Verification items for the finished model (mm, model axes). Face numbers are marked on the shaded views. A direction names the side the tool comes from. Coordinates: 2 decimals unless noted, no trailing zeros. Loops run counter-clockwise (first coordinate to the right, second up) from the corner with the lowest first, then second, coordinate; pieces in that order, holes last. Notation, with made-up numbers: (-4, 86.25) -> (23, 86.25) arc R22 ccw to (23, 92.25) -> close; hole circle Ø1 at (-23.5, -7.75). An arc over 180 degrees is marked (long way). Use CSV: the item, a comma, the result in double quotes. Start each with the question number.
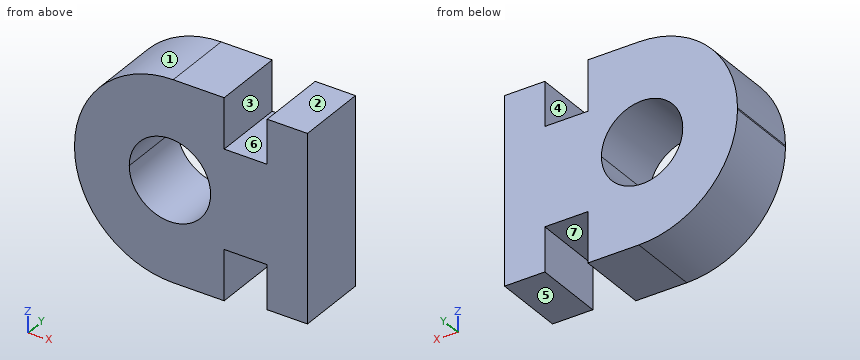
```python
from build123d import *

# Parameters (mm, degrees)
F1_DEPTH = 28.956
F2_R     = 39.858666


with BuildPart() as f1:
    # F0 (on Front) → F1 (new body)
    with BuildSketch(Plane.XZ):
        with BuildLine():
            Line((0, -37.671965), (0, 0))
            Line((0, 0), (-39.146767, 0))
            ThreePointArc((-39.146767, 0), (-55.584025, -16.437258), (-72.021282, 0))
            Line((-72.021282, 0), (-94.127469, 0))
            Line((-94.127469, 0), (-94.127469, -40.149245))
            Line((-94.127469, -40.149245), (-65.204445, -40.149245))
            Line((-65.204445, -40.149245), (-55.504855, -40.149245))
            Line((-55.504855, -40.149245), (-33.65957, -40.149245))
            Line((-33.65957, -40.149245), (-33.65957, -19.839078))
            Line((-33.65957, -19.839078), (-16.272509, -19.839078))
            Line((-16.272509, -19.839078), (-16.272509, -36.780316))
            Line((-16.272509, -36.780316), (-16.272509, -37.671965))
            Line((-16.272509, -37.671965), (0, -37.671965))
        make_face()
        with BuildLine():
            Line((0, 0), (0, 37.671965))
            Line((0, 37.671965), (-16.272509, 37.671965))
            Line((-16.272509, 37.671965), (-16.272509, 36.780316))
            Line((-16.272509, 36.780316), (-16.272509, 19.839078))
            Line((-16.272509, 19.839078), (-33.65957, 19.839078))
            Line((-33.65957, 19.839078), (-33.65957, 40.149245))
            Line((-33.65957, 40.149245), (-55.504855, 40.149245))
            Line((-55.504855, 40.149245), (-65.204445, 40.149245))
            Line((-65.204445, 40.149245), (-94.127469, 40.149245))
            Line((-94.127469, 40.149245), (-94.127469, 0))
            Line((-94.127469, 0), (-72.021282, 0))
            ThreePointArc((-72.021282, 0), (-55.584025, 16.437258), (-39.146767, 0))
            Line((-39.146767, 0), (0, 0))
        make_face()
    extrude(amount=F1_DEPTH)

    # F2
    f2_edges = [f1.edges().sort_by_distance(p)[0] for p in [
        (-94.127469, -14.478, 40.149245),
        (-94.127469, -14.478, -40.149245),
    ]]
    fillet(f2_edges, radius=F2_R)


solid = f1.part
```
1. Cross-section at A-A, the plane z = -28.5. Record the boundary of the cut face in (x, y), plus the area to 3 significant figures.
2. Cross-section at B-B, the plane y = -3.5. Record the boundary of the cut face in (x, z).
3. Release check for a two-part mould opening along X. For the marked faces 1, 2, 3 and 4 record: released by +X, released by -X, zero draft, split by the parting line, or undercut.
4. Scan lines: line 1 (X direction, y = -16.5, z = -25); line 2 (X direction, y = -6.75, z = 15); line 3 (Z direction, x = -45.5, y = -23.5). Record each from-to range of solid material in increasing order.
5. Cross-section at D-D, the plane x = -28.5. Record the boundary of the cut face in (y, z).
6. Depth check by flat-ended pin: pin 1 (3 mm diameter, centred on y = -20.5, z = -28.5, fed in from -X); pin 2 (8 mm diameter, centred on y = -17.5, z = -16, fed in from -X); pin 3 (1.5 mm diameter, centred on x = -76.5, y = -8.5, fed in from +Z). Enter the tip coordinate at first touch or a pass-through.
7. Set-up check for the marked faces 5, 6 and 7: record each of +Z, -Z, +X, -X, +Y, -Y from which the full face is reachable in a straight line by a thin tool's end or side.
8. Cross-section at C-C, the plane x = -61. Record the boundary of the cut face in (y, z), plus the area to 3 significant figures.
Solution:
1,outline,"(-82.43, -28.96) -> (-33.66, -28.96) -> (-33.66, 0) -> (-82.43, 0) -> close; (-16.27, -28.96) -> (0, -28.96) -> (0, 0) -> (-16.27, 0) -> close"
1,area,"1,880 mm2"
2,outline,"(-94.13, -0.29) arc R39.86 ccw to (-54.27, -40.15) -> (-33.66, -40.15) -> (-33.66, -19.84) -> (-16.27, -19.84) -> (-16.27, -37.67) -> (0, -37.67) -> (0, 37.67) -> (-16.27, 37.67) -> (-16.27, 19.84) -> (-33.66, 19.84) -> (-33.66, 40.15) -> (-54.27, 40.15) arc R39.86 ccw to (-94.13, 0.29) -> close; hole circle Ø32.87 at (-55.58, 0)"
3,face 1,"released by -X"
3,face 2,"zero draft"
3,face 3,"undercut"
3,face 4,"undercut"
4,line 1,"x = -85.54 to -33.66, -16.27 to 0"
4,line 2,"x = -91.31 to -62.31, -48.86 to 0"
4,line 3,"z = -40.15 to -12.98, 12.98 to 40.15"
5,outline,"(-28.96, -19.84) -> (0, -19.84) -> (0, 19.84) -> (-28.96, 19.84) -> close"
6,pin 1,"stops at x = -83.85"
6,pin 2,"stops at x = -92.37"
6,pin 3,"stops at z = 33.87"
7,face 5,"-Z, +X, +Y, -Y"
7,face 6,"+Z, +Y, -Y"
7,face 7,"-Z, +Y, -Y"
8,outline,"(-28.96, -39.58) -> (0, -39.58) -> (0, -15.52) -> (-28.96, -15.52) -> close; (-28.96, 15.52) -> (0, 15.52) -> (0, 39.58) -> (-28.96, 39.58) -> close"
8,area,"1,390 mm2"
